Can you work these out from the model? Positions are in its coordinate system, mm. Face numbers are marked on the shaded views. A direction names the side the tool comes from. Round coordinates to 2 decimals unless told otherwise and drop trailing zeros. Order: outer loops, then holes, each group sorted by start corner. A loop starts at its lowest first (then second) coordinate and runs counter-clockwise, first axis right, second up. Notation, with made-up numbers: M 50.25,-10.75 L 63.25,-10.75 A16 ccw 63.25,-2.75 Z; hole C 26.5,14.25 d2. An arc over 180 degrees is marked long. One line per question, with ' | ' between items.
Solid Edge part; units mm, degrees
sketch "Sketch1" plane through (0, 0, -8.3) normal (0, 0, 1) x (1, 0, 0)
  circle A0 centre (-7.5, -6.25) radius 2.2
  circle A1 centre (12.5, -6.25) radius 2.2
  circle A2 centre (12.5, 6.25) radius 2.2
  line L0 (-13, 10.75) -> (18, 10.75)
  line L1 (18, 10.75) -> (18, -10.75)
  line L2 (18, -10.75) -> (-13, -10.75)
  line L3 (-13, -10.75) -> (-13, 10.75)
  circle A3 centre (-7.5, 6.25) radius 2.2
  dimension "D1" = 13
  dimension "D2" = 18
extrude "Protrusion1" add sketch "Sketch1" along normal up to vertex (8.3 mm away)
sketch "Sketch2" plane through (2.5, 18.75, -4.15) normal (1, 0, 0) x (0, 1, 0)
  line L0 (-11.2268, -4.15) -> (-14.9595, 2.3153)
  line L1 (-14.9595, 2.3153) -> (-22.5405, 2.3153)
  line L2 (-22.5405, 2.3153) -> (-26.2732, -4.15)
extrude "ExtrudedCutout_1" cut sketch "Sketch2" along normal mid plane 6.4 material side at (2.5, 5.6135, -5.0923)
sketch "Sketch3" plane through (18, 18.75, -4.15) normal (1, 0, 0) x (0, -1, 0)
  circle A0 centre (18.75, 4.15) radius 5
extrude "Cutout1" cut sketch "Sketch3" against normal through all
sketch "Sketch4" plane through (2.5, 7.875, -8.3) normal (0, 0, -1) x (-1, 0, 0)
  line L0 (-12.2, -1.625) -> (-12.2, -14.125)
  line L1 (-7.8, -14.125) -> (-7.8, -1.625)
  arc A0 (-7.8, -14.125) -> (-12.2, -14.125) centre (-10, -14.125) ccw
  arc A1 (-7.8, -1.625) -> (-12.2, -1.625) centre (-10, -1.625) cw
  line L2 (7.8, -1.625) -> (7.8, -14.125)
  arc A2 (12.2, -14.125) -> (7.8, -14.125) centre (10, -14.125) cw
  line L3 (12.2, -14.125) -> (12.2, -1.625)
  arc A3 (12.2, -1.625) -> (7.8, -1.625) centre (10, -1.625) ccw
extrude "ExtrudedCutout_4" cut sketch "Sketch4" against normal blind 3.5
properties material "ABS Plastic, medium impact"
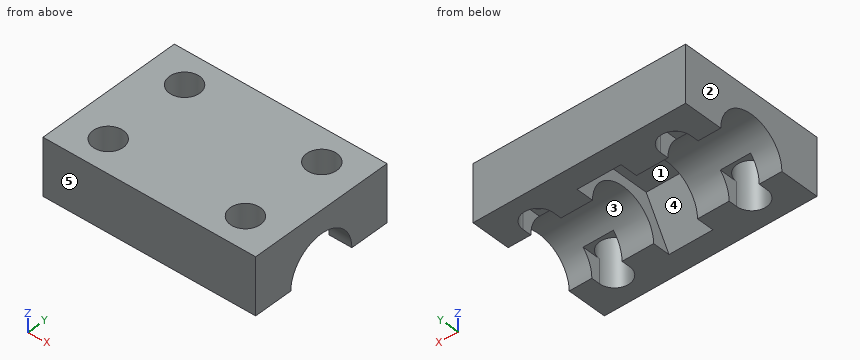
(1) If we section it at B-B on z = -1.5: Please give me the cut outline in (x, y).
Final values:
outline: M -13,-10.75 L 18,-10.75 L 18,10.75 L -13,10.75 Z; hole C -7.5,-6.25 d4.4; hole C -7.5,6.25 d4.4; hole C 12.5,-6.25 d4.4; hole C 12.5,6.25 d4.4
(2) On a 3-axis mill with a long thin cutter (end or side, diameter ignored), from which of +Z, -Z, +X, -X, +Y, -Y can I reach the whole of each face in a straight line? I mean the marked faces 4 and 5. Say none if no direction works.
Final values:
face 4: -Z | face 5: +Z, -Z, +X, -X, -Y
(3) Will this pin go through, and if not, where does the flat tip stop? pin 1 Ø3 at (x, y) = (-8, 5.5) entering from -Z.
Final values:
pin 1: z = -4.8
(4) If we section it at D-D on y = 0: Please give me the cut outline in (x, z), plus the area to 3 significant figures.
Final values:
outline: M -13,-3.3 L -0.7,-3.3 L -0.7,-1.83 L 5.7,-1.83 L 5.7,-3.3 L 18,-3.3 L 18,0 L -13,0 Z | area: 92.9 mm^2
(5) Please list where these lines run through material, in increasing order: probe 1 along X at (y, z) = (6.25, -2.25); probe 2 along Y at (x, z) = (-7.5, -1.75); probe 3 along X at (y, z) = (2.25, -3.5). Write a range as [from, to].
Final values:
probe 1: [-13, -9.7], [-5.3, 10.3], [14.7, 18] | probe 2: [-10.75, -8.45], [-4.05, 4.05], [8.45, 10.75] | probe 3: [-13, -0.7], [5.7, 18]
(6) If we section it at A-A on x = 12.5: Please give me the cut outline in (y, z).
Final values:
outline: M -10.75,-8.3 L -8.45,-8.3 L -8.45,0 L -10.75,0 Z; M -4.05,-4.8 L -3.57,-4.8 A5 cw 3.57,-4.8 L 4.05,-4.8 L 4.05,0 L -4.05,0 Z; M 8.45,-8.3 L 10.75,-8.3 L 10.75,0 L 8.45,0 Z
(7) Thinking about a two-plate mould opening in X: for the marked faces 1, 2 and 3, which applies, released by +X, released by -X, zero draft, split by the parting line, or undercut?
Final values:
face 1: undercut | face 2: released by -X | face 3: zero draft
